from build123d import *

# Parameters (mm, degrees)
SKETCH1_R           = 4.75
GEAR_ROOT_DEPTH     = 6
SKETCH3_R           = 1
NEEDLE_SHAFT_DEPTH  = 18
BOSS_EXTRUDE1_DEPTH = 6
SKETCH7_R           = 0.6
CUT_EXTRUDE1_DEPTH  = 10


with BuildPart() as part:
    # Sketch1 → GEAR_ROOT (new body)
    with BuildSketch(Plane(origin=(0, 0, 0), x_dir=(1, 0, 0), z_dir=(0, 1, 0))):
        with Locations(Location((0, 0, 0), (0, 0, 270))):
            Circle(SKETCH1_R)
    extrude(amount=GEAR_ROOT_DEPTH)

    # Sketch3 → NEEDLE_SHAFT (add)
    with BuildSketch(Plane(origin=(0, 0, 0), x_dir=(1, 0, 0), z_dir=(0, 1, 0))):
        with Locations(Location((0, 0, 0), (0, 0, 270))):
            Circle(SKETCH3_R)
    extrude(amount=NEEDLE_SHAFT_DEPTH)

    # Sketch6 → Boss-Extrude1 (add)
    with BuildSketch(Plane.XZ):
        with BuildLine():
            Line((0.61, 6.95761567), (-0.61, 6.95761567))
            Line((-0.61, 6.95761567), (-0.786402192, 4.684449978))
            ThreePointArc((-0.786402192, 4.684449978), (0, 4.75), (0.786402192, 4.684449978))
            Line((0.786402192, 4.684449978), (0.61, 6.95761567))
        make_face()
        with BuildLine():
            Line((4.583084249, 5.270280314), (3.596083516, 5.987378321))
            Line((3.596083516, 5.987378321), (2.117237874, 4.252035252))
            ThreePointArc((2.117237874, 4.252035252), (2.791979948, 3.842830723), (3.38966335, 3.32756403))
            Line((3.38966335, 3.32756403), (4.583084249, 5.270280314))
        make_face()
        with BuildLine():
            Line((6.805586088, 1.569877008), (6.428585355, 2.730165957))
            Line((6.428585355, 2.730165957), (4.212165035, 2.195487582))
            ThreePointArc((4.212165035, 2.195487582), (4.517518452, 1.467830723), (4.698188318, 0.699661723))
            Line((4.698188318, 0.699661723), (6.805586088, 1.569877008))
        make_face()
        with BuildLine():
            Line((6.428585355, -2.730165957), (6.805586088, -1.569877008))
            Line((6.805586088, -1.569877008), (4.698188318, -0.699661723))
            ThreePointArc((4.698188318, -0.699661723), (4.517518452, -1.467830723), (4.212165035, -2.195487582))
            Line((4.212165035, -2.195487582), (6.428585355, -2.730165957))
        make_face()
        with BuildLine():
            Line((3.596083516, -5.987378321), (4.583084249, -5.270280314))
            Line((4.583084249, -5.270280314), (3.38966335, -3.32756403))
            ThreePointArc((3.38966335, -3.32756403), (2.791979948, -3.842830723), (2.117237874, -4.252035252))
            Line((2.117237874, -4.252035252), (3.596083516, -5.987378321))
        make_face()
        with BuildLine():
            Line((-0.61, -6.95761567), (0.61, -6.95761567))
            Line((0.61, -6.95761567), (0.786402192, -4.684449978))
            ThreePointArc((0.786402192, -4.684449978), (0, -4.75), (-0.786402192, -4.684449978))
            Line((-0.786402192, -4.684449978), (-0.61, -6.95761567))
        make_face()
        with BuildLine():
            Line((-4.583084249, -5.270280314), (-3.596083516, -5.987378321))
            Line((-3.596083516, -5.987378321), (-2.117237874, -4.252035252))
            ThreePointArc((-2.117237874, -4.252035252), (-2.791979948, -3.842830723), (-3.38966335, -3.32756403))
            Line((-3.38966335, -3.32756403), (-4.583084249, -5.270280314))
        make_face()
        with BuildLine():
            Line((-6.805586088, -1.569877008), (-6.428585355, -2.730165957))
            Line((-6.428585355, -2.730165957), (-4.212165035, -2.195487582))
            ThreePointArc((-4.212165035, -2.195487582), (-4.517518452, -1.467830723), (-4.698188318, -0.699661723))
            Line((-4.698188318, -0.699661723), (-6.805586088, -1.569877008))
        make_face()
        with BuildLine():
            Line((-6.428585355, 2.730165957), (-6.805586088, 1.569877008))
            Line((-6.805586088, 1.569877008), (-4.698188318, 0.699661723))
            ThreePointArc((-4.698188318, 0.699661723), (-4.517518452, 1.467830723), (-4.212165035, 2.195487582))
            Line((-4.212165035, 2.195487582), (-6.428585355, 2.730165957))
        make_face()
        with BuildLine():
            Line((-3.596083516, 5.987378321), (-4.583084249, 5.270280314))
            Line((-4.583084249, 5.270280314), (-3.38966335, 3.32756403))
            ThreePointArc((-3.38966335, 3.32756403), (-2.791979948, 3.842830723), (-2.117237874, 4.252035252))
            Line((-2.117237874, 4.252035252), (-3.596083516, 5.987378321))
        make_face()
    extrude(amount=-BOSS_EXTRUDE1_DEPTH)

    # Sketch7 → Cut-Extrude1 (cut)
    with BuildSketch(Plane(origin=(1.228784274, 0, 0.860284377), x_dir=(0.5735229177482851, 0, -0.8191895158127294), z_dir=(0.8191895158127294, 0, 0.5735229177482851))):
        with Locations((0, 15.53461336)):
            Circle(SKETCH7_R)
    extrude(amount=-CUT_EXTRUDE1_DEPTH, mode=Mode.SUBTRACT)


solid = part.part
Geometry: final body of the model. Coordinates: model frame, mm. A direction names the side the tool comes from. Coordinates: 2 decimals unless noted, no trailing zeros. Loops run counter-clockwise (first coordinate to the right, second up) from the corner with the lowest first, then second, coordinate; pieces in that order, holes last. Notation, with made-up numbers: (4, 88.25) - (40, 88.25) arc R26 ccw to (40, 110.25) - close; hole circle Ø5 at (9.5, -18). An arc over 180 degrees is marked (long way). One line per question, with ' | ' between items. Start each with the question number.
(1) First-contact query: pin 1 (1 mm diameter, centred on y = 2, z = 4, fed in from +X); pin 2 (1.5 mm diameter, centred on x = 4.5, z = 3.5, fed in from +Y); pin 3 (4 mm diameter, centred on x = -4.5, z = -1, fed in from +Y); pin 4 (1.5 mm diameter, centred on y = 7.5, z = -1.5, fed in from +X). Flat tips, straight axial feed; report the tip coordinate or a pass-through.
(2) Cut plane A-A on x = 5.25. Output: boundary loops of the cut face in (y, z), and give its area (3 significant figures).
(3) Draft query along X for faces 6 (the cylindrical face through (-0.33, 15.56, 0.5)), 7 (the flat face through (-5.767, 2.958, 1.141)), 8 (the flat face through (3.98, 2.96, 4.29)), 9 (the cylindrical face through (1.477, 2.958, -4.514)). Return one class per face: +X half, -X half, draft (parallel to the pull), parting line (faces both ways), or undercut.
(4) Ray query, L1, parallel to X at y = 3, z = -5.25; L2, parallel to X at y = 2.75, z = 4.75; L3, parallel to Z at x = 0, y = 14.5. Return the intervals inside material, ascending. Write a range as from..to.
(5) Cut plane B-B on y = 14. Output: boundary loops of the cut face in (x, z), and give its area (3 significant figures).
(6) Cut plane C-C on z = 4. Output: boundary loops of the cut face in (x, y), and give its area (3 significant figures).
(7) Cut plane D-D on x = 1.75. Output: boundary loops of the cut face in (y, z).
(8) Reachability of faces 1 (the flat face through (-5.74, 2.96, -1.13)), 2 (the flat face through (-2.867, 2.958, -5.132)), 3 (the cylindrical face through (3.837, 2.958, 2.8)), 4 (the flat face through (3.995, 2.958, -4.313)), 5 (the flat face through (-2.85, 2.96, 5.11)) from +Z, -Z, +X, -X, +Y, -Y: full face, straight path, thin tool, end or side. Return the list, or none.
Here are the results:
1) pin 1: x = 4.11 | pin 2: through | pin 3: y = 6 | pin 4: x = 0.66
2) outline: (0, -2.45) - (6, -2.45) - (6, -0.93) - (0, -0.93) - close; (0, 0.93) - (6, 0.93) - (6, 2.45) - (0, 2.45) - close | area: 18.2 mm²
3) face 6: undercut | face 7: -X half | face 8: +X half | face 9: undercut
4) L1: -4.57..-2.97, -0.74..0.74, 2.97..4.57 | L2: -4.26..-2.54, -0.78..0.78, 2.54..4.26 | L3: -1..1
5) outline: circle Ø2 at (0, 0) | area: 3.14 mm²
6) outline: (-3.8, 0) - (3.8, 0) - (3.8, 6) - (-3.8, 6) - close | area: 45.6 mm²
7) outline: (0, -4.42) - (6, -4.42) - (6, 4.42) - (0, 4.42) - close
8) face 1: -X, +Y, -Y | face 2: -Z, +Y, -Y | face 3: +Y, -Y | face 4: +X, +Y, -Y | face 5: +Z, +Y, -Y
